Answer from the drawing. Dimensions are ordinates in mm from the lowest x, y and z of the part. A direction names the side the tool comes from. Give positions to 0.01 mm unless a question says otherwise; leave off trailing zeros. Order: outer loops, then holes, each group sorted by start corner. A loop starts at its lowest first (then second) coordinate and runs counter-clockwise, first axis right, second up.
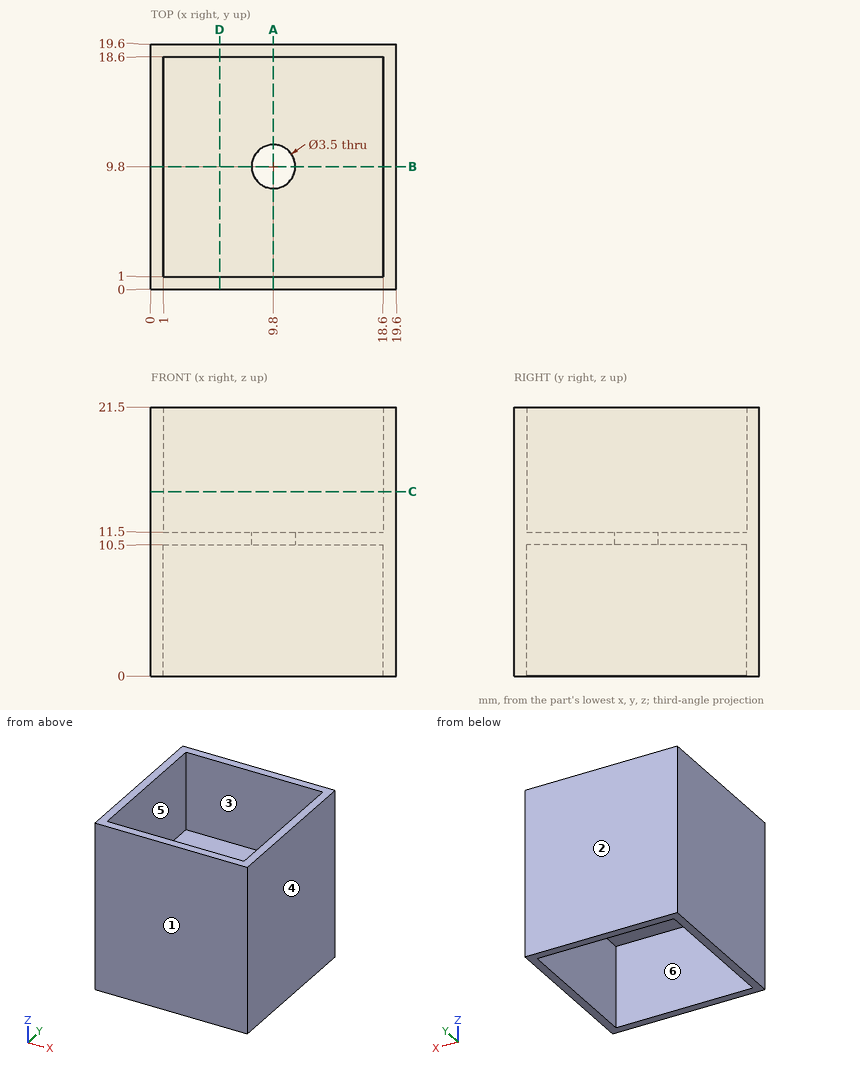
1. The mould has two halves that part along Y. Classify the marked faces 1, 2 and 3: pulls with the +Y half, pulls with the -Y half, needs draft (parallel to the pull), parting line crosses it, or undercut.
Findings below:
face 1: pulls with the -Y half
face 2: pulls with the +Y half
face 3: undercut
2. Which of the six approach directions +Z, -Z, +X, -X, +Y, -Y give full straight-line access (tool end or side, diameter ignored) to the marked faces 4, 5 and 6?
Findings below:
face 4: +Z, -Z, +X, +Y, -Y
face 5: +Z
face 6: -Z
3. The part is cut by section A-A (x = 9.8). Write down the section's boundary in (y, z), then the cut area to 3 significant figures.
Findings below:
outline: (0, 0) - (1, 0) - (1, 10.5) - (8.05, 10.5) - (8.05, 11.5) - (1, 11.5) - (1, 21.5) - (0, 21.5) - close; (11.55, 10.5) - (18.6, 10.5) - (18.6, 0) - (19.6, 0) - (19.6, 21.5) - (18.6, 21.5) - (18.6, 11.5) - (11.55, 11.5) - close
area: 57.1 mm2
4. Given P1, Ø3, axis at x = 9.8, y = 9.8, coming from the -Z side; P2, Ø9, axis at x = 10, y = 13.5, coming from the -Z side; P3, Ø4, axis at x = 11.5, y = 5, coming from the +Z side, each flat-ended and moving along its own axis, determine where each tip first touches the part or whether it passes through.
Findings below:
P1: passes through
P2: stops at z = 10.5
P3: stops at z = 11.5
5. The part is cut by section C-C (z = 14.75). Write down the section's boundary in (x, y).
Findings below:
outline: (0, 0) - (19.6, 0) - (19.6, 19.6) - (0, 19.6) - close; hole (1, 1) - (18.6, 1) - (18.6, 18.6) - (1, 18.6) - close
6. The part is cut by section D-D (x = 5.5). Write down the section's boundary in (y, z).
Findings below:
outline: (0, 0) - (1, 0) - (1, 10.5) - (18.6, 10.5) - (18.6, 0) - (19.6, 0) - (19.6, 21.5) - (18.6, 21.5) - (18.6, 11.5) - (1, 11.5) - (1, 21.5) - (0, 21.5) - close
7. Straight lines are drawn through the part: probe 1 along Y at (x, z) = (5, 10.25); probe 2 along Y at (x, z) = (9.8, 10.8). For each, find the intervals that lie inside material, in ascending order.
Findings below:
probe 1: y = 0 to 1, 18.6 to 19.6
probe 2: y = 0 to 8.05, 11.55 to 19.6
